from build123d import *

# Parameters (mm, degrees)
POCKET004_DEPTH = 1
SKETCH013_R     = 1
PAD005_DEPTH    = 12.7


with BuildPart() as part:
    # Sketch011 → Revolution001 (revolve)
    with BuildSketch(Plane.XZ):
        with BuildLine():
            Line((0, 0), (0, 1.5748))
            Line((0, 1.5748), (0.5, 1.5748))
            ThreePointArc((2.1209, 0.5), (1.472434, 1.281687), (0.5, 1.5748))
            Line((2.1209, 0.5), (2.1209, 0))
            Line((2.1209, 0), (0, 0))
        make_face()
    revolve(axis=Axis((0, 0, 0), (0, 0, 1)))

    # Sketch012 (on Face1 of Revolution001) → Pocket004 (cut)
    with BuildSketch(Plane(origin=(0, 0, 1.5748), x_dir=(-1, 0, 0), z_dir=(0, 0, 1))):
        with BuildLine():
            ThreePointArc((0.375, 1), (0, 1.375), (-0.375, 1))
            Line((-0.375, 1), (-0.375, 0.375))
            Line((-0.375, 0.375), (-1, 0.375))
            ThreePointArc((-1, 0.375), (-1.375, 0), (-1, -0.375))
            Line((-1, -0.375), (-0.375, -0.375))
            Line((-0.375, -0.375), (-0.375, -1))
            ThreePointArc((-0.375, -1), (0, -1.375), (0.375, -1))
            Line((0.375, -1), (0.375, -0.375))
            Line((0.375, -0.375), (1, -0.375))
            ThreePointArc((1, -0.375), (1.375, 0), (1, 0.375))
            Line((1, 0.375), (0.375, 0.375))
            Line((0.375, 0.375), (0.375, 1))
        make_face()
    extrude(amount=-POCKET004_DEPTH, mode=Mode.SUBTRACT)

    # Sketch013 (on Face16 of Pocket004) → Pad005 (join)
    with BuildSketch(Plane(origin=(0, 0, 0), x_dir=(1, 0, 0), z_dir=(0, 0, -1))):
        Circle(SKETCH013_R)
    extrude(amount=PAD005_DEPTH)


with BuildPart() as part_1:
    # Body003 placement: moved
    add(part.part.moved(Location((14, 7, 7.75))))


solid = part_1.part
Verification items for the finished model (mm, model axes). A direction names the side the tool comes from. Coordinates: 2 decimals unless noted, no trailing zeros. Order: outer loops, then holes, each group sorted by start corner. A loop starts at its lowest first (then second) coordinate and runs counter-clockwise, first axis right, second up. Notation, with made-up numbers: M -15,63.5 L 1,63.5 A17 ccw 1,73.5 Z; hole C 82,55 d1. An arc over 180 degrees is marked long. One line per item, written item: value. Start each with the question number.
Item 1: Sectioned sample at B-B (z = -3.25). Enter the section's corners in (x, y).
Item 2: Sectioned sample at A-A (z = 8). Enter the section's corners in (x, y), then the cut area to 3 significant figures.
Item 3: Gauge pin test, flat ends, axial feed: pin 1 (1 mm diameter, centred on x = 14, z = -0.5, fed in from -Y); pin 2 (2 mm diameter, centred on x = 13, y = 7.5, fed in from +Z); pin 3 (0.5 mm diameter, centred on y = 6, z = 8.5, fed in from -X); pin 4 (0.7 mm diameter, centred on x = 13.5, z = 8.5, fed in from +Y). Record the tip position at first contact, or that the pin passes through.
Item 4: Access from +Z, -Z, +X, -X, +Y, -Y to the whole of each face (thin tool, end or side, straight path). Record for faces 1 (the flat face through (14, 7, -4.95)), 2 (the flat face through (14, 7, 8.325)), 3 (the flat face through (13, 6, 7.75)).
Item 5: Scan lines: probe 1 along Z at (x, y) = (13.8, 7.25); probe 2 along Y at (x, z) = (14.4, -3.25); probe 3 along Z at (x, y) = (14.5, 8.7). Record each from-to range of solid material in increasing order.
Conclusion:
1. outline: C 14,7 d2
2. outline: C 14,7 d4.24
2. area: 14.1 mm^2
3. pin 1: stops at y = 6
3. pin 2: stops at z = 9.32
3. pin 3: stops at x = 12.08
3. pin 4: stops at y = 9.11
4. face 1: -Z, +X, -X, +Y, -Y
4. face 2: +Z
4. face 3: -Z
5. probe 1: z = -4.95 to 8.32
5. probe 2: y = 6.08 to 7.92
5. probe 3: z = 7.75 to 8.78
